Could you check a few things on this model? Use its own coordinates, in mm. Face numbers are marked on the shaded views. A direction names the side the tool comes from. Give positions to 0.01 mm unless a question says otherwise; leave off trailing zeros. Order: outer loops, then holes, each group sorted by start corner. A loop starts at its lowest first (then second) coordinate and runs counter-clockwise, first axis right, second up. Notation, with made-up numbers: (6, 23) - (19, 23) arc R28 cw to (19, 53) - close; hole circle Ø2 at (33, 42.5). An arc over 180 degrees is marked (long way). One line per question, with ' | ' between items. Start each with the question number.
1. Imagine slicing it at D-D (x = -12). Please give me the cut outline in (y, z), and give its area (3 significant figures).
2. Imagine slicing it at B-B (z = 5.5). Give the number of separate pieces and of enclosed holes in the cut face, and give its area (3 significant figures).
3. Imagine slicing it at C-C (y = -38.1). Please give me the cut outline in (x, z).
4. Imagine slicing it at A-A (y = -68). Please give me the cut outline in (x, z), and give its area (3 significant figures).
5. If we mould it in two halves opening along Y, with no side actions, what happens to the marked faces 1, 2, 3 and 4? For each: released by +Y, released by -Y, zero draft, split by the parting line, or undercut.
6. Which directions (+Z, -Z, +X, -X, +Y, -Y) give clear straight access to the entire face, cutting with the end or side of a thin tool? Please do the marked faces 5 and 6.
7. For P1, Ø2, axis at x = -19, z = 6.5, coming from the -Y side; P2, Ø1.5, axis at x = 12.15, y = -12.38, coming from the -Z side; P3, Ø2.5, axis at y = -16.5, z = 5.5, coming from the -X side; P4, Ø1, axis at y = -19, z = 8, coming from the -X side, each with a flat end and sliding along its axis, tell me the tip position at first contact or that it passes through.
8. I need wall thicknesses on probe 1 along Y at (x, z) = (35.5, 1.75) (3 decimals); probe 2 along Y at (x, z) = (11.5, 5.5) (3 decimals); probe 3 along X at (y, z) = (-45, 2.5). Which ranges of each line are inside material? Lowest first, please. Write a range as from..to.
```python
from build123d import *

# Parameters (mm, degrees)
BOSS_EXTRUDE1_DEPTH      = 8.89
SKETCH9_R                = 1.267511842
SKETCH9_W                = 3.81
SKETCH9_H                = 8.128
SKETCH9_W_2              = 3.556
SKETCH9_H_2              = 13.97
SKETCH9_W_3              = 8.73125
SKETCH9_H_3              = 3.96875
CUT_EXTRUDE6_DEPTH       = 1
CUT_EXTRUDE6_DEPTH_BACK  = 9.89
SKETCH4_W                = 34.29
SKETCH4_H                = 30.48
CUT_EXTRUDE7_DEPTH       = 7.9375
CUT_EXTRUDE7_DEPTH_BACK  = 1
SKETCH3_R                = 5.08
CUT_EXTRUDE8_DEPTH       = 1
CUT_EXTRUDE8_DEPTH_BACK  = 9.89
SKETCH12_R               = 1.27
CUT_EXTRUDE9_DEPTH       = 1
CUT_EXTRUDE9_DEPTH_BACK  = 9.89
SKETCH15_R               = 1.27
CUT_EXTRUDE10_DEPTH      = 1
CUT_EXTRUDE10_DEPTH_BACK = 9.89


with BuildPart() as part:
    # Sketch1 → Boss-Extrude1 (new body)
    with BuildSketch(Plane.XY):
        with BuildLine():
            Line((-3.314058103, 6.35), (48.26, 6.35))
            ThreePointArc((48.26, 6.35), (51.852102448, 4.862102448), (53.34, 1.27))
            Line((53.34, 1.27), (53.34, -92.71))
            ThreePointArc((53.34, -92.71), (51.852102448, -96.302102448), (48.26, -97.79))
            Line((48.26, -97.79), (16.846989059, -97.79))
            ThreePointArc((16.846989059, -97.79), (15.638688158, -97.644208035), (14.499741809, -97.215200367))
            Line((14.499741809, -97.215200367), (-16.7505185, -80.933552139))
            ThreePointArc((-16.7505185, -80.933552139), (-18.059258376, -79.955412607), (-18.989802686, -78.61241436))
            Line((-18.989802686, -78.61241436), (-28.309569459, -59.040904135))
            ThreePointArc((-28.309569459, -59.040904135), (-28.795802898, -57.127870198), (-28.51617555, -55.173917704))
            Line((-28.51617555, -55.173917704), (-8.107195629, 2.952923842))
            ThreePointArc((-8.107195629, 2.952923842), (-6.251501454, 5.414614163), (-3.314058103, 6.35))
        make_face()
    extrude(amount=BOSS_EXTRUDE1_DEPTH)

    # Sketch9 → Cut-Extrude6 (cut, two sides)
    with BuildSketch(Plane(origin=(0, 0, 0), x_dir=(-1, 0, 0), z_dir=(0, 0, -1))) as cut_extrude6_sk:
        with Locations((-5.348417946, -30.953529248)):
            Circle(SKETCH9_R)
        with Locations((-32.218986844, -9.676052932)):
            Circle(SKETCH9_R)
        with Locations((-12.150498686, -12.37729109)):
            Circle(SKETCH9_R)
        with Locations((-12.150498686, -26.66479109)):
            Circle(SKETCH9_R)
        with Locations((-28.057248686, -12.37729109)):
            Circle(SKETCH9_R)
        with Locations((-5.348417946, -9.676052932)):
            Circle(SKETCH9_R)
        with Locations((-32.218986844, -30.953529248)):
            Circle(SKETCH9_R)
        with Locations((-28.057248686, -26.66479109)):
            Circle(SKETCH9_R)
        with Locations((-10.245904396, -20.31479109)):
            Rectangle(SKETCH9_W, SKETCH9_H)
        Polygon((-15.064842187, -33.01479109), (-23.802748686, -33.01479109), (-23.802748686, -26.66479109), (-20.913498686, -26.66479109), (-15.064842187, -26.66479109), align=None)
        with Locations((-35.010498686, -19.798068783)):
            Rectangle(SKETCH9_W_2, SKETCH9_H_2)
        with Locations((-19.310123686, -9.59916609)):
            Rectangle(SKETCH9_W_3, SKETCH9_H_3)
    extrude(amount=CUT_EXTRUDE6_DEPTH, mode=Mode.SUBTRACT)
    extrude(cut_extrude6_sk.sketch, amount=-CUT_EXTRUDE6_DEPTH_BACK, mode=Mode.SUBTRACT)

    # Sketch4 → Cut-Extrude7 (cut, two sides)
    with BuildSketch(Plane.XY) as cut_extrude7_sk:
        with Locations((20.024498686, -18.415)):
            Rectangle(SKETCH4_W, SKETCH4_H)
    extrude(amount=CUT_EXTRUDE7_DEPTH, mode=Mode.SUBTRACT)
    extrude(cut_extrude7_sk.sketch, amount=-CUT_EXTRUDE7_DEPTH_BACK, mode=Mode.SUBTRACT)

    # Sketch3 → Cut-Extrude8 (cut, two sides)
    with BuildSketch(Plane.XY.offset(8.89)) as cut_extrude8_sk:
        with Locations((3.878385852, -38.1)):
            Circle(SKETCH3_R)
        with Locations((-5.011614148, -46.99)):
            Circle(SKETCH3_R)
        with Locations((3.878385852, -55.88)):
            Circle(SKETCH3_R)
        with Locations((12.768385852, -46.99)):
            Circle(SKETCH3_R)
        with Locations((-9.144, -65.024)):
            Circle(SKETCH3_R)
        with Locations((3.048, -70.612)):
            Circle(SKETCH3_R)
        with Locations((15.24, -76.2)):
            Circle(SKETCH3_R)
    extrude(amount=CUT_EXTRUDE8_DEPTH, mode=Mode.SUBTRACT)
    extrude(cut_extrude8_sk.sketch, amount=-CUT_EXTRUDE8_DEPTH_BACK, mode=Mode.SUBTRACT)

    # Sketch12 → Cut-Extrude9 (cut, two sides)
    with BuildSketch(Plane(origin=(0, 0, 0), x_dir=(-1, 0, 0), z_dir=(0, 0, -1))) as cut_extrude9_sk:
        with Locations((-48.0822, 2.286)):
            Circle(SKETCH12_R)
        with Locations((3.718687848, 1.651)):
            Circle(SKETCH12_R)
        with Locations((25.012261453, -59.761967182)):
            Circle(SKETCH12_R)
    extrude(amount=CUT_EXTRUDE9_DEPTH, mode=Mode.SUBTRACT)
    extrude(cut_extrude9_sk.sketch, amount=-CUT_EXTRUDE9_DEPTH_BACK, mode=Mode.SUBTRACT)

    # Sketch15 → Cut-Extrude10 (cut, two sides)
    with BuildSketch(Plane(origin=(0, 0, 0), x_dir=(-1, 0, 0), z_dir=(0, 0, -1))) as cut_extrude10_sk:
        with Locations((18.034, -57.15)):
            Circle(SKETCH15_R)
        with Locations((-43.942, -85.852)):
            Circle(SKETCH15_R)
    extrude(amount=CUT_EXTRUDE10_DEPTH, mode=Mode.SUBTRACT)
    extrude(cut_extrude10_sk.sketch, amount=-CUT_EXTRUDE10_DEPTH_BACK, mode=Mode.SUBTRACT)


solid = part.part
```
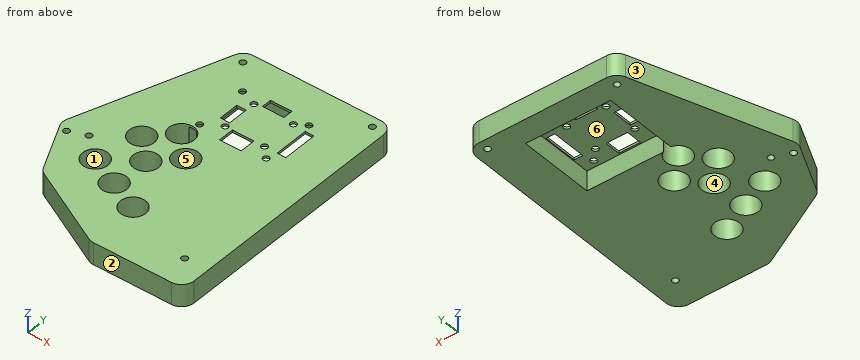
Results found:
1) outline: (-83.41, 0) - (-69.23, 0) - (-69.23, 8.89) - (-83.41, 8.89) - close; (-60.82, 0) - (-8.13, 0) - (-8.13, 8.89) - (-60.82, 8.89) - close | area: 594 mm2
2) separate pieces: 1 | enclosed holes: 12 | area: 5,620 mm2
3) outline: (-22.52, 0) - (-1.2, 0) - (-1.2, 8.89) - (-22.52, 8.89) - close; (8.96, 0) - (53.34, 0) - (53.34, 8.89) - (8.96, 8.89) - close
4) outline: (-24.04, 0) - (-13.26, 0) - (-13.26, 8.89) - (-24.04, 8.89) - close; (-5.03, 0) - (-1.31, 0) - (-1.31, 8.89) - (-5.03, 8.89) - close; (7.41, 0) - (53.34, 0) - (53.34, 8.89) - (7.41, 8.89) - close | area: 537 mm2
5) face 1: undercut | face 2: released by -Y | face 3: released by +Y | face 4: undercut
6) face 5: +Z, -Z | face 6: -Z
7) P1: stops at y = -80.02 | P2: passes through | P3: stops at x = -15.38 | P4: stops at x = -15.99
8) probe 1: y = -97.79..-33.655, -3.175..6.35 | probe 2: y = -95.652..-79.638, -72.762..-51.909, -42.071..-33.655, -3.175..6.35 | probe 3: x = -24.94..-9.69, -0.34..8.09, 17.44..53.34
